Geometry: final body of the model. Coordinates: model frame, mm. Face numbers are marked on the shaded views. A direction names the side the tool comes from. Round coordinates to 2 decimals unless told otherwise and drop trailing zeros. Write each loop counter-clockwise with the first axis right and the second up, starting at its lowest first coordinate (ties: lowest second). Pieces come first, ordered by that corner, then holes. Notation, with made-up numbers: M -17,-39 L 27,-39 A19 cw 27,-3 Z; hole C 82,15.5 d5. An arc over 180 degrees is marked long. Use one line per item in the form item = value. Start each with the question number.
Item 1: Ray query, probe 1 along X at (y, z) = (19.3, 72); probe 2 along Y at (x, z) = (-81, 23); probe 3 along X at (y, z) = (28.75, 40.5). Return the intervals inside material, ascending.
Item 2: Pin query (flat end, axial travel): pin 1 Ø5 at (x, z) = (-49.16, 72) entering from -Y; pin 2 Ø6 at (x, y) = (-73, 42) entering from +Z; pin 3 Ø0.6 at (y, z) = (18.5, 43.5) entering from -X; pin 4 Ø5 at (y, z) = (30, 37.5) entering from +X. Return the tip coordinate at first contact, or that it passes through.
Item 3: Section query C-C (y = 27.5). Return loops of the section in (x, z).
Item 4: Section query A-A (z = 57). Return loops of the section in (x, y), and give its area (3 significant figures).
Item 5: Reachability of the marked faces 1, 2, 3 and 4 from +Z, -Z, +X, -X, +Y, -Y: full face, straight path, thin tool, end or side. Return the list, or none.
Item 6: Section query B-B (x = -85). Return loops of the section in (y, z), and give its area (3 significant figures).
Item 7: Section query D-D (z = -3). Return loops of the section in (x, y), and give its area (3 significant figures).
Item 8: Pull-direction query (Z, two-part tool) for the marked faces 5, 6 and 7; classes: pulls with the +Z half, pulls with the -Z half, needs draft (parallel to the pull), parting line crosses it, or undercut.
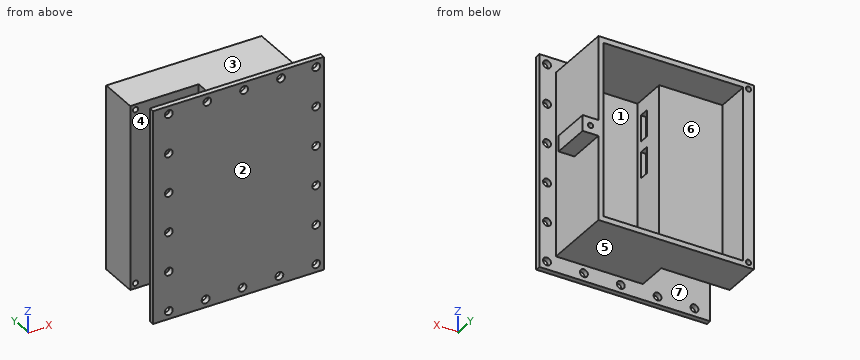
from build123d import *

# Parameters (mm, degrees)
BOSS_EXTRU_1_DEPTH                  = 70
ESQUISSE2_W                         = 64.879929842
ESQUISSE2_H                         = 80.999999972
ESQUISSE2_R                         = 1.499999992
ESQUISSE2_R_2                       = 1.499999996
ESQUISSE2_R_3                       = 1.499999991
ESQUISSE2_R_4                       = 1.499999993
ESQUISSE2_R_5                       = 1.499999999
ESQUISSE2_R_6                       = 1.5
BOSS_EXTRU_2_DEPTH                  = 2
COQUE1_START                        = 19.900521193
COQUE1_OUTLINE_W                    = 29
COQUE1_OUTLINE_H                    = 66
COQUE1_DEPTH                        = 26.5
COQUE1_START_2                      = 33.400521193
COQUE1_2_OUTLINE_W                  = 24
COQUE1_2_OUTLINE_H                  = 66
COQUE1_2_DEPTH                      = 13
ENL_V_MAT_EXTRU_1_REACH             = 98.547
ESQUISSE4_W                         = 10
ESQUISSE4_H                         = 4
ENL_V_MAT_EXTRU_2_REACH             = 98.547
ESQUISSE5_W                         = 10
ESQUISSE5_H                         = 4
ESQUISSE8_W                         = 70
ESQUISSE8_H                         = 15
BOSS_EXTRU_4_DEPTH                  = 2
ENL_V_MAT_EXTRU_4_REACH             = 128.81
ESQUISSE9_R                         = 1
ENL_V_MAT_EXTRU_4_DIRECTION_2_DEPTH = 127.809653192
ESQUISSE10_W                        = 6
ESQUISSE10_H                        = 15
BOSS_EXTRU_5_DEPTH                  = 6
ESQUISSE11_R                        = 1
ENL_V_MAT_EXTRU_5_DEPTH             = 21


# Read off the part's stored shape, not the designer's step: Coque1
with BuildPart() as part:
    # Esquisse1 → Boss.-Extru.1 (new body)
    with BuildSketch(Plane.XY):
        Polygon((-96.201008889, 46.400521193), (-39.201008889, 46.400521193), (-39.201008889, 19.900521193), (-72.201008889, 19.900521193), (-72.201008889, 31.400521193), (-96.201008889, 31.400521193), align=None)
    extrude(amount=BOSS_EXTRU_1_DEPTH)

    # Esquisse2 → Boss.-Extru.2 (add)
    with BuildSketch(Plane(origin=(0, 19.900521193, 0), x_dir=(-1, 0, 0), z_dir=(0, -1, 0))):
        with Locations((65.355645606, -34.499999986)):
            Rectangle(ESQUISSE2_W, ESQUISSE2_H)
        with Locations(Location((35.797436273, -71.999999972, 0), (0, 0, 180))):
            Circle(ESQUISSE2_R, mode=Mode.SUBTRACT)
        with Locations(Location((35.797290063, -56.999999973, 0), (0, 0, 180))):
            Circle(ESQUISSE2_R_2, mode=Mode.SUBTRACT)
        with Locations(Location((35.797008085, -41.999999976, 0), (0, 0, 180))):
            Circle(ESQUISSE2_R_3, mode=Mode.SUBTRACT)
        with Locations(Location((35.796726108, -26.999999979, 0), (0, 0, 180))):
            Circle(ESQUISSE2_R_4, mode=Mode.SUBTRACT)
        with Locations(Location((35.796274405, -11.999999985, 0), (0, 0, 180))):
            Circle(ESQUISSE2_R_5, mode=Mode.SUBTRACT)
        with Locations(Location((35.795610527, 3, 0), (0, 0, 180))):
            Circle(ESQUISSE2_R_6, mode=Mode.SUBTRACT)
        with Locations(Location((49.795610527, 3, 0), (0, 0, 180))):
            Circle(ESQUISSE2_R_6, mode=Mode.SUBTRACT)
        with Locations(Location((63.795610527, 3, 0), (0, 0, 180))):
            Circle(ESQUISSE2_R_6, mode=Mode.SUBTRACT)
        with Locations(Location((77.795610527, 3, 0), (0, 0, 180))):
            Circle(ESQUISSE2_R_6, mode=Mode.SUBTRACT)
        with Locations(Location((91.795610527, 3, 0), (0, 0, 180))):
            Circle(ESQUISSE2_R_6, mode=Mode.SUBTRACT)
        with Locations(Location((91.795610527, -12, 0), (0, 0, 180))):
            Circle(ESQUISSE2_R_6, mode=Mode.SUBTRACT)
        with Locations(Location((91.795610527, -27, 0), (0, 0, 180))):
            Circle(ESQUISSE2_R_6, mode=Mode.SUBTRACT)
        with Locations(Location((91.795610527, -42, 0), (0, 0, 180))):
            Circle(ESQUISSE2_R_6, mode=Mode.SUBTRACT)
        with Locations(Location((91.795610527, -57, 0), (0, 0, 180))):
            Circle(ESQUISSE2_R_6, mode=Mode.SUBTRACT)
        with Locations(Location((91.795610527, -72, 0), (0, 0, 180))):
            Circle(ESQUISSE2_R_6, mode=Mode.SUBTRACT)
        with Locations(Location((49.163080617, -71.999999972, 0), (0, 0, 180))):
            Circle(ESQUISSE2_R, mode=Mode.SUBTRACT)
        with Locations(Location((63.163080617, -71.999999972, 0), (0, 0, 180))):
            Circle(ESQUISSE2_R, mode=Mode.SUBTRACT)
        with Locations(Location((77.163080617, -71.999999972, 0), (0, 0, 180))):
            Circle(ESQUISSE2_R, mode=Mode.SUBTRACT)
    extrude(amount=BOSS_EXTRU_2_DEPTH)

    # Coque1 outline → Coque1 (cut)
    with BuildSketch(Plane(origin=(0, 0, 0), x_dir=(1, 0, 0), z_dir=(0, 1, 0)).offset(COQUE1_START)):
        with Locations((-55.701008889, -35)):
            Rectangle(COQUE1_OUTLINE_W, COQUE1_OUTLINE_H)
    extrude(amount=COQUE1_DEPTH, mode=Mode.SUBTRACT)

    # Coque1 2 outline → Coque1 2 (cut)
    with BuildSketch(Plane(origin=(0, 0, 0), x_dir=(1, 0, 0), z_dir=(0, 1, 0)).offset(COQUE1_START_2)):
        with Locations((-82.201008889, -35)):
            Rectangle(COQUE1_2_OUTLINE_W, COQUE1_2_OUTLINE_H)
    extrude(amount=COQUE1_2_DEPTH, mode=Mode.SUBTRACT)

    # Esquisse4 → Enlèv. mat.-Extru.1 (cut, up to next)
    with BuildSketch(Plane.ZY.offset(72.201008889), mode=Mode.PRIVATE) as enl_v_mat_extru_1_sk1:
        with Locations((57.5, 23.900521193)):
            Rectangle(ESQUISSE4_W, ESQUISSE4_H)
    enl_v_mat_extru_1_tool1 = extrude(enl_v_mat_extru_1_sk1.sketch, amount=-ENL_V_MAT_EXTRU_1_REACH, mode=Mode.PRIVATE) & part.part
    add(enl_v_mat_extru_1_tool1.solids().sort_by_distance((-72.201009, 23.900521, 57.5))[0], mode=Mode.SUBTRACT)

    # Esquisse5 → Enlèv. mat.-Extru.2 (cut, up to next)
    with BuildSketch(Plane.ZY.offset(72.201008889), mode=Mode.PRIVATE) as enl_v_mat_extru_2_sk1:
        with Locations((43.5, 23.900521193)):
            Rectangle(ESQUISSE5_W, ESQUISSE5_H)
    enl_v_mat_extru_2_tool1 = extrude(enl_v_mat_extru_2_sk1.sketch, amount=-ENL_V_MAT_EXTRU_2_REACH, mode=Mode.PRIVATE) & part.part
    add(enl_v_mat_extru_2_tool1.solids().sort_by_distance((-72.201009, 23.900521, 43.5))[0], mode=Mode.SUBTRACT)

    # Esquisse8 → Boss.-Extru.4 (add)
    with BuildSketch(Plane.ZY.offset(96.201008889)):
        with Locations((35, 38.900521193)):
            Rectangle(ESQUISSE8_W, ESQUISSE8_H)
    extrude(amount=BOSS_EXTRU_4_DEPTH)

    # Esquisse9 → Enlèv. mat.-Extru.4 (cut, up to next)
    with BuildSketch(Plane(origin=(0, 46.400521193, 0), x_dir=(1, 0, 0), z_dir=(0, 1, 0)), mode=Mode.PRIVATE) as enl_v_mat_extru_4_sk1:
        with Locations(Location((-96.201008889, -2, 0), (0, 0, 90))):
            Circle(ESQUISSE9_R)
    enl_v_mat_extru_4_tool1 = extrude(enl_v_mat_extru_4_sk1.sketch, amount=-ENL_V_MAT_EXTRU_4_REACH, mode=Mode.PRIVATE) & part.part
    # Esquisse9 → Enlèv. mat.-Extru.4 (cut, up to next)
    with BuildSketch(Plane(origin=(0, 46.400521193, 0), x_dir=(1, 0, 0), z_dir=(0, 1, 0)), mode=Mode.PRIVATE) as enl_v_mat_extru_4_sk2:
        with Locations(Location((-96.201008889, -68, 0), (0, 0, 90))):
            Circle(ESQUISSE9_R)
    enl_v_mat_extru_4_tool2 = extrude(enl_v_mat_extru_4_sk2.sketch, amount=-ENL_V_MAT_EXTRU_4_REACH, mode=Mode.PRIVATE) & part.part
    add(enl_v_mat_extru_4_tool1.solids().sort_by_distance((-96.201009, 46.400521, 2))[0], mode=Mode.SUBTRACT)
    add(enl_v_mat_extru_4_tool2.solids().sort_by_distance((-96.201009, 46.400521, 68))[0], mode=Mode.SUBTRACT)

    # Esquisse9 → Enlèv. mat.-Extru.4 direction 2 (cut)
    with BuildSketch(Plane(origin=(0, 46.400521193, 0), x_dir=(1, 0, 0), z_dir=(0, 1, 0))):
        with Locations(Location((-96.201008889, -2, 0), (0, 0, 90))):
            Circle(ESQUISSE9_R)
        with Locations(Location((-96.201008889, -68, 0), (0, 0, 90))):
            Circle(ESQUISSE9_R)
    extrude(amount=ENL_V_MAT_EXTRU_4_DIRECTION_2_DEPTH, mode=Mode.SUBTRACT)

    # Esquisse10 → Boss.-Extru.5 (add)
    with BuildSketch(Plane(origin=(-39.201008889, 0, 0), x_dir=(0, 0, -1), z_dir=(1, 0, 0))):
        with Locations((-35, 38.900521193)):
            Rectangle(ESQUISSE10_W, ESQUISSE10_H)
    extrude(amount=BOSS_EXTRU_5_DEPTH)

    # Esquisse11 → Enlèv. mat.-Extru.5 (cut)
    with BuildSketch(Plane(origin=(0, 46.400521193, 0), x_dir=(1, 0, 0), z_dir=(0, 1, 0))):
        with Locations(Location((-36.201008889, -35, 0), (0, 0, 270))):
            Circle(ESQUISSE11_R)
    extrude(amount=-ENL_V_MAT_EXTRU_5_DEPTH, mode=Mode.SUBTRACT)


solid = part.part
Working result:
q1.probe_1 = -97.8 to -93.3, -90.3 to -78.66, -75.66 to -64.66, -61.66 to -50.66, -47.66 to -37.3, -34.3 to -32.92
q1.probe_2 = 17.9 to 19.9, 31.4 to 33.4
q1.probe_3 = -72.2 to -70.2, -41.2 to -39.2
q2.pin_1 = 17.9
q2.pin_2 = 70
q2.pin_3 = -97.8
q2.pin_4 = -33.2
q3.outline = M -72.2,0 L -39.2,0 L -39.2,70 L -72.2,70 Z; hole M -70.2,2 L -41.2,2 L -41.2,68 L -70.2,68 Z
q4.outline = M -98.2,31.4 L -72.2,31.4 L -72.2,25.9 L -70.2,25.9 L -70.2,33.4 L -94.2,33.4 L -94.2,46.4 L -98.2,46.4 Z; M -97.8,17.9 L -93.3,17.9 L -93.3,19.9 L -97.8,19.9 Z; M -90.3,17.9 L -37.3,17.9 L -37.3,19.9 L -39.2,19.9 L -39.2,46.4 L -41.2,46.4 L -41.2,19.9 L -70.2,19.9 L -70.2,21.9 L -72.2,21.9 L -72.2,19.9 L -90.3,19.9 Z; M -34.3,17.9 L -32.92,17.9 L -32.92,19.9 L -34.3,19.9 Z
q4.area = 294 mm²
q5.face_1 = +Y
q5.face_2 = +Z, -Z, +X, -X, -Y
q5.face_3 = +Z, +X, -X, +Y
q5.face_4 = +Z, -Z, -X
q6.outline = M 17.9,-6 L 19.9,-6 L 19.9,75 L 17.9,75 Z; M 31.4,0 L 46.4,0 L 46.4,2 L 33.4,2 L 33.4,68 L 46.4,68 L 46.4,70 L 31.4,70 Z
q6.area = 354 mm²
q7.outline = M -97.8,17.9 L -93.3,17.9 L -93.3,19.9 L -97.8,19.9 Z; M -90.3,17.9 L -79.3,17.9 L -79.3,19.9 L -90.3,19.9 Z; M -76.3,17.9 L -65.3,17.9 L -65.3,19.9 L -76.3,19.9 Z; M -62.3,17.9 L -51.3,17.9 L -51.3,19.9 L -62.3,19.9 Z; M -48.3,17.9 L -37.3,17.9 L -37.3,19.9 L -48.3,19.9 Z; M -34.3,17.9 L -32.92,17.9 L -32.92,19.9 L -34.3,19.9 Z
q7.area = 99.8 mm²
q8.face_5 = pulls with the -Z half
q8.face_6 = undercut
q8.face_7 = needs draft
